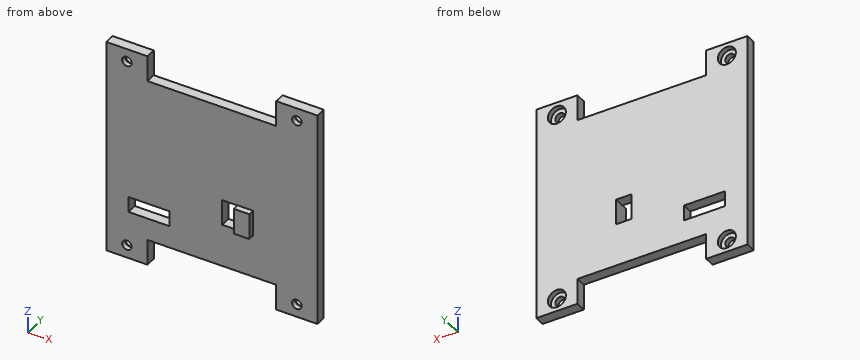
from build123d import *

# Parameters (mm, degrees)
SKETCH1_W           = 35
SKETCH1_H           = 26
BOSS_EXTRUDE1_DEPTH = 2
SKETCH2_W           = 41
SKETCH2_H           = 32
BOSS_EXTRUDE3_DEPTH = 2
SKETCH4_W           = 8
SKETCH4_H           = 2
BOSS_EXTRUDE4_DEPTH = 5
SKETCH5_W           = 8
SKETCH5_H           = 2
BOSS_EXTRUDE5_DEPTH = 5
SKETCH6_R           = 0.925
CUT_EXTRUDE1_DEPTH  = 5
SKETCH7_R           = 1.75
CUT_EXTRUDE2_DEPTH  = 1
SKETCH8_W           = 3
SKETCH8_H           = 5
BOSS_EXTRUDE6_DEPTH = 1.2
SKETCH9_W           = 3
SKETCH9_H           = 4.959490372
SKETCH9_W_2         = 8
SKETCH9_H_2         = 3
CUT_EXTRUDE3_DEPTH  = 2


with BuildPart() as part:
    # Sketch1 → Boss-Extrude1 (new body)
    with BuildSketch(Plane(origin=(0, 0, 0), x_dir=(1, 0, 0), z_dir=(0, 1, 0))):
        with Locations((4.316901408, -0.671361502)):
            Rectangle(SKETCH1_W, SKETCH1_H)
    extrude(amount=BOSS_EXTRUDE1_DEPTH)

    # Sketch2 → Boss-Extrude3 (add)
    with BuildSketch(Plane(origin=(0, 2, 0), x_dir=(1, 0, 0), z_dir=(0, 1, 0))):
        with Locations((4.316901408, -0.671361502)):
            Rectangle(SKETCH2_W, SKETCH2_H)
    extrude(amount=-BOSS_EXTRUDE3_DEPTH)

    # Sketch4 → Boss-Extrude4 (add)
    with BuildSketch(Plane(origin=(0, 0, -15.328638498), x_dir=(-1, 0, 0), z_dir=(0, 0, -1))):
        with Locations((12.183098592, 1)):
            Rectangle(SKETCH4_W, SKETCH4_H)
        with Locations((-20.816901408, 1)):
            Rectangle(SKETCH4_W, SKETCH4_H)
    extrude(amount=BOSS_EXTRUDE4_DEPTH)

    # Sketch5 → Boss-Extrude5 (add)
    with BuildSketch(Plane.XY.offset(16.671361502)):
        with Locations((20.816901408, 1)):
            Rectangle(SKETCH5_W, SKETCH5_H)
        with Locations((-12.183098592, 1)):
            Rectangle(SKETCH5_W, SKETCH5_H)
    extrude(amount=BOSS_EXTRUDE5_DEPTH)

    # Sketch6 → Cut-Extrude1 (cut)
    with BuildSketch(Plane(origin=(0, 2, 0), x_dir=(1, 0, 0), z_dir=(0, 1, 0))):
        with Locations((-12.183098592, 17.828638498)):
            Circle(SKETCH6_R)
        with Locations((20.816901408, 17.828638498)):
            Circle(SKETCH6_R)
        with Locations((20.816901408, -19.171361502)):
            Circle(SKETCH6_R)
        with Locations((-12.183098592, -19.171361502)):
            Circle(SKETCH6_R)
    extrude(amount=-CUT_EXTRUDE1_DEPTH, mode=Mode.SUBTRACT)

    # Sketch7 → Cut-Extrude2 (cut)
    with BuildSketch(Plane(origin=(0, 2, 0), x_dir=(1, 0, 0), z_dir=(0, 1, 0))):
        with Locations((-12.183098592, 17.828638498)):
            Circle(SKETCH7_R)
        with Locations((20.816901408, 17.828638498)):
            Circle(SKETCH7_R)
        with Locations((20.816901408, -19.171361502)):
            Circle(SKETCH7_R)
        with Locations((-12.183098592, -19.171361502)):
            Circle(SKETCH7_R)
    extrude(amount=-CUT_EXTRUDE2_DEPTH, mode=Mode.SUBTRACT)

    # Sketch8 → Boss-Extrude6 (add)
    with BuildSketch(Plane.XZ):
        with Locations((10.816901408, -4.528382577)):
            Rectangle(SKETCH8_W, SKETCH8_H)
    extrude(amount=BOSS_EXTRUDE6_DEPTH)

    # Sketch9 → Cut-Extrude3 (cut)
    with BuildSketch(Plane.XZ):
        with Locations((7.816901408, -4.548637391)):
            Rectangle(SKETCH9_W, SKETCH9_H)
        with Locations((-7.857851807, -9.519264119)):
            Rectangle(SKETCH9_W_2, SKETCH9_H_2)
    extrude(amount=-CUT_EXTRUDE3_DEPTH, mode=Mode.SUBTRACT)


solid = part.part
Geometry: final body of the model. Coordinates: model frame, mm. Give positions to 0.01 mm unless a question says otherwise; leave off trailing zeros. Write each loop counter-clockwise with the first axis right and the second up, starting at its lowest first coordinate (ties: lowest second). Pieces come first, ordered by that corner, then holes. Notation, with made-up numbers: (21.5, -14.75) -> (46.5, -14.75) arc R8 ccw to (46.5, -5.75) -> close; hole circle Ø8 at (43, 36.25). An arc over 180 degrees is marked (long way). Answer as a JSON object with one key per item and string values.
1. Cut plane D-D on x = 5.5. Output: boundary loops of the cut face in (y, z), and give its area (3 significant figures).
Ans:
{"outline": "(0, -15.33) -> (2, -15.33) -> (2, 16.67) -> (0, 16.67) -> close", "area": "64.0 mm^2"}
2. Cut plane A-A on x = -5. Output: boundary loops of the cut face in (y, z), and give its area (3 significant figures).
Ans:
{"outline": "(0, -15.33) -> (2, -15.33) -> (2, -11.02) -> (0, -11.02) -> close; (0, -8.02) -> (2, -8.02) -> (2, 16.67) -> (0, 16.67) -> close", "area": "58.0 mm^2"}
3. Contact query for flat-ended pins moving along their axis: pin 1 (1.6 mm diameter, centred on x = 8.5, y = 0.5, fed in from -Z); pin 2 (1.8 mm diameter, centred on x = -13, z = -18.5, fed in from +Y); pin 3 (1.5 mm diameter, centred on x = -0.5, z = -9.5, fed in from -Y); pin 4 (0.6 mm diameter, centred on x = 4.5, y = 1.5, fed in from +Z). Output: stop coordinate, or through.
Ans:
{"pin 1": "stops at z = -15.33", "pin 2": "stops at y = 2", "pin 3": "stops at y = 0", "pin 4": "stops at z = 16.67"}
4. Cut plane C-C on y = -0.65. Output: boundary loops of the cut face in (x, z).
Ans:
{"outline": "(9.32, -7.03) -> (12.32, -7.03) -> (12.32, -2.03) -> (9.32, -2.03) -> close"}
5. Ray query, probe 1 along Z at (x, y) = (-12, 0.2); probe 2 along X at (y, z) = (0.6, -6); probe 3 along X at (y, z) = (0.1, -8.5). Return the intervals inside material, ascending. Write a range as from..to.
Ans:
{"probe 1": "z = -20.33..-18.74, -16.92..18.26, 20.08..21.67", "probe 2": "x = -16.18..6.32, 9.32..24.82", "probe 3": "x = -16.18..-11.86, -3.86..24.82"}
6. Cut plane B-B on z = -3. Output: boundary loops of the cut face in (x, y).
Ans:
{"outline": "(-16.18, 0) -> (6.32, 0) -> (6.32, 2) -> (-16.18, 2) -> close; (9.32, -1.2) -> (12.32, -1.2) -> (12.32, 0) -> (24.82, 0) -> (24.82, 2) -> (9.32, 2) -> close"}
